Could you check a few things on this drawing? It's one solid part, dimensions in mm from its lowest x, y, z. Give positions to 0.01 mm unless a question says otherwise; leave off trailing zeros. Loops run counter-clockwise (first coordinate to the right, second up) from the corner with the lowest first, then second, coordinate; pieces in that order, holes last.
Q1. Suppose I cut it at C-C (x = 171.45). List the corners of the cut face in (y, z) for me, and give its area (3 significant figures).
Q2. Suppose I cut it at D-D (z = 1.25). Count the separate pieces of the cut face and the enclosed holes in it, and give its area (3 significant figures).
Q3. I need wall thicknesses on probe 1 along Y at (x, z) = (6.35, 2); probe 2 along X at (y, z) = (12.5, 1.75) (1 decimal); probe 3 along X at (y, z) = (7, 0.5) (1 decimal). Which ranges of each line are inside material? Lowest first, please.
Q4. I'm going to push a flat-ended pin straight in: P1, Ø10, axis at x = 130.12, y = 11.86, coming from the -Z side. Where does the tip first touch, or does it pass through?
Q5. Suppose I cut it at A-A (x = 88.9). List the corners of the cut face in (y, z) for me, and give its area (3 significant figures).
Q6. Suppose I cut it at B-B (y = 31.75). List the corners of the cut face in (x, z) for me.
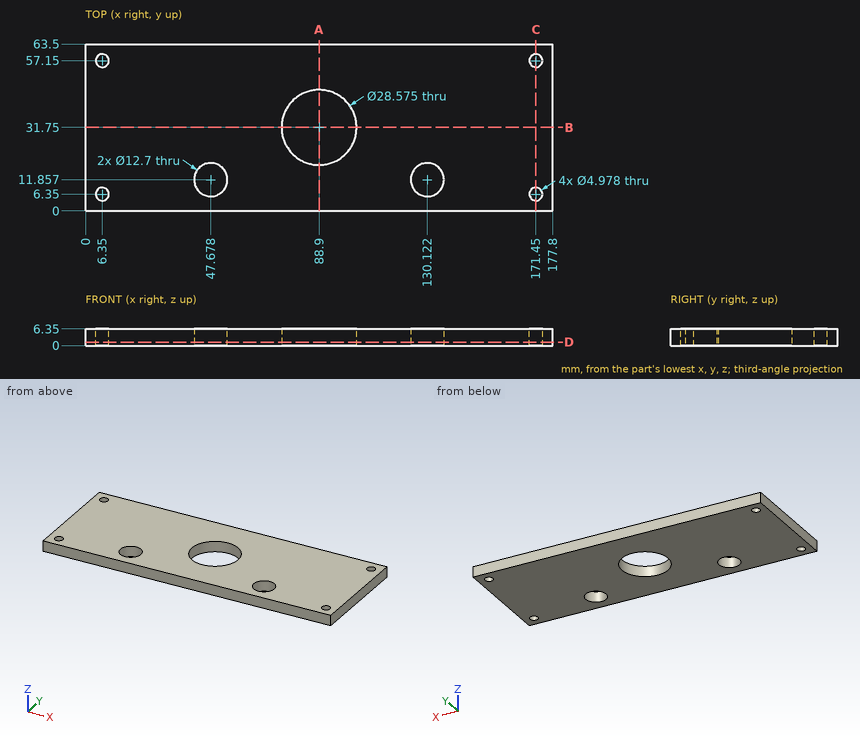
Solutions:
1. outline: (0, 0) - (3.86, 0) - (3.86, 6.35) - (0, 6.35) - close; (8.84, 0) - (54.66, 0) - (54.66, 6.35) - (8.84, 6.35) - close; (59.64, 0) - (63.5, 0) - (63.5, 6.35) - (59.64, 6.35) - close
1. area: 340 mm2
2. separate pieces: 1
2. enclosed holes: 7
2. area: 10,300 mm2
3. probe 1: y = 0 to 3.86, 8.84 to 54.66, 59.64 to 63.5
3. probe 2: x = 0 to 41.4, 54 to 123.8, 136.4 to 177.8
3. probe 3: x = 0 to 3.9, 8.8 to 43.6, 51.8 to 126, 134.2 to 169, 173.9 to 177.8
4. P1: passes through
5. outline: (0, 0) - (17.46, 0) - (17.46, 6.35) - (0, 6.35) - close; (46.04, 0) - (63.5, 0) - (63.5, 6.35) - (46.04, 6.35) - close
5. area: 222 mm2
6. outline: (0, 0) - (74.61, 0) - (74.61, 6.35) - (0, 6.35) - close; (103.19, 0) - (177.8, 0) - (177.8, 6.35) - (103.19, 6.35) - close
